Solid Edge part; units mm, degrees
sketch "Sketch1" plane through (0, 0, 0) normal (0, 0, 1) x (1, 0, 0)
  line L0 (-22.5, -10) -> (22.5, -10)
  line L1 (22.5, -10) -> (22.5, 10)
  line L2 (22.5, 10) -> (-22.5, 10)
  line L3 (-22.5, 10) -> (-22.5, -10)
extrude "Protrusion1" add sketch "Sketch1" along normal blind 1.5
sketch "Sketch2" plane through (0, 0, 1.5) normal (0, 0, 1) x (1, 0, 0)
  circle A0 centre (-13, 0) radius 8
  circle A1 centre (13, 0) radius 8
extrude "ultrasone" add sketch "Sketch2" along normal blind 12
hole "Hole_1" at (-13, 0, 13.5) direction (0, 0, -1) diameter 14 depth 1
hole "Hole1" at (13, 0, 13.5) direction (0, 0, -1) diameter 14 depth 1
The listing builds one solid part. Answer for the finished solid, in the listing's coordinates (mm). A direction names the side the tool comes from. Give positions to 0.01 mm unless a question says otherwise; leave off trailing zeros. Write each loop counter-clockwise with the first axis right and the second up, starting at its lowest first coordinate (ties: lowest second). Pieces come first, ordered by that corner, then holes.
1) For a pull along Y with two mould halves and no side action, classify faces 3 (the face through (-14.73, 7.81, 7.42)), 4 (the face through (-9, -6, 13.5)), 5 (the face through (13, 0, 12.5)) as pulls with the +Y half, pulls with the -Y half, needs draft (parallel to the pull), parting line crosses it, or undercut.
2) Section D-D (x = 9.5) is taken. Write down the section's boundary in (y, z).
3) Section A-A (y = 0) is taken. Write down the section's boundary in (x, z), and give its area (4 significant figures).
4) Given P1, Ø8, axis at y = 3.5, z = 6.5, coming from the +X side; P2, Ø2, axis at x = 6, z = 11, coming from the -Y side; P3, Ø10, axis at x = 1.5, y = -1.5, coming from the +Z side; P4, Ø4, axis at x = -11.5, y = -0.5, coming from the +Z side, each flat-ended and moving along its own axis, determine where each tip first touches the part or whether it passes through.
5) A tool of negligible diameter and unlimited length cuts with its end or side. For faces 1 (the face through (-22.5, 0, 1)), 2 (the face through (11.27, 7.81, 7.42)), from which of +Z, -Z, +X, -X, +Y, -Y can it reach the whole face along a straight path? Write none if from no direction.
6) Section B-B (x = -13) is taken. Write down the section's boundary in (y, z).
7) Find the intervals of material crossed by L1, parallel to Y at x = 13, z = 13.2; L2, parallel to Z at x = 12, y = 9; L3, parallel to Z at x = 10, y = -6, in increasing order.
8) Section C-C (z = 6.25) is taken. Write down the section's boundary in (x, y).
Response:
1. face 3: parting line crosses it
1. face 4: needs draft
1. face 5: undercut
2. outline: (-10, 0) - (10, 0) - (10, 1.5) - (7.19, 1.5) - (7.19, 13.5) - (6.06, 13.5) - (6.06, 12.5) - (-6.06, 12.5) - (-6.06, 13.5) - (-7.19, 13.5) - (-7.19, 1.5) - (-10, 1.5) - close
3. outline: (-22.5, 0) - (22.5, 0) - (22.5, 1.5) - (21, 1.5) - (21, 13.5) - (20, 13.5) - (20, 12.5) - (6, 12.5) - (6, 13.5) - (5, 13.5) - (5, 1.5) - (-5, 1.5) - (-5, 13.5) - (-6, 13.5) - (-6, 12.5) - (-20, 12.5) - (-20, 13.5) - (-21, 13.5) - (-21, 1.5) - (-22.5, 1.5) - close
3. area: 423.5 mm2
4. P1: stops at x = 21
4. P2: stops at y = -5.29
4. P3: stops at z = 13.5
4. P4: stops at z = 12.5
5. face 1: +Z, -Z, -X, +Y, -Y
5. face 2: +Z
6. outline: (-10, 0) - (10, 0) - (10, 1.5) - (8, 1.5) - (8, 13.5) - (7, 13.5) - (7, 12.5) - (-7, 12.5) - (-7, 13.5) - (-8, 13.5) - (-8, 1.5) - (-10, 1.5) - close
7. L1: y = -8 to -7, 7 to 8
7. L2: z = 0 to 1.5
7. L3: z = 0 to 12.5
8. outline: circle Ø16 at (-13, 0); circle Ø16 at (13, 0)
